Check sheet for the drawn part. Datum: minimum x, y, z corner. Units: mm. A direction names the side the tool comes from. Give positions to 0.01 mm unless a question says otherwise; leave off trailing zeros. Loops run counter-clockwise (first coordinate to the right, second up) from the corner with the lowest first, then second, coordinate; pieces in that order, holes last. Notation, with made-up numbers: (41, -15.5) - (54, -15.5) arc R19 cw to (54, 11.5) - close; hole circle Ø10 at (63, 46). An arc over 180 degrees is marked (long way). One line per item, written item: value. Start each with the question number.
1. Gauge pin test, flat ends, axial feed: pin 1 (5.5 mm diameter, centred on x = 6, z = 3.5, fed in from +Y); pin 2 (4 mm diameter, centred on x = 2.5, z = 47.5, fed in from +Y); pin 3 (5 mm diameter, centred on x = 6.5, y = 22.5, fed in from -Z); pin 4 (3 mm diameter, centred on y = 18, z = 25, fed in from +X). Record the tip position at first contact, or that the pin passes through.
2. Sectioned sample at A-A (z = 25). Record the cut outline in (x, y), plus the area to 3 significant figures.
3. Scan lines: L1, parallel to Y at x = 5, z = 25; L2, parallel to Y at x = 2, z = 39; L3, parallel to Y at x = 7, z = 2. Record each from-to range of solid material in increasing order. Write a range as [from, to].
4. Sectioned sample at C-C (y = 19.75). Record the cut outline in (x, z), plus the area to 3 significant figures.
5. Access from +Z, -Z, +X, -X, +Y, -Y to the whole of each face (thin tool, end or side, straight path). Record for the marked faces 1, 2 and 3.
6. Sectioned sample at D-D (z = 4.5). Record the cut outline in (x, y).
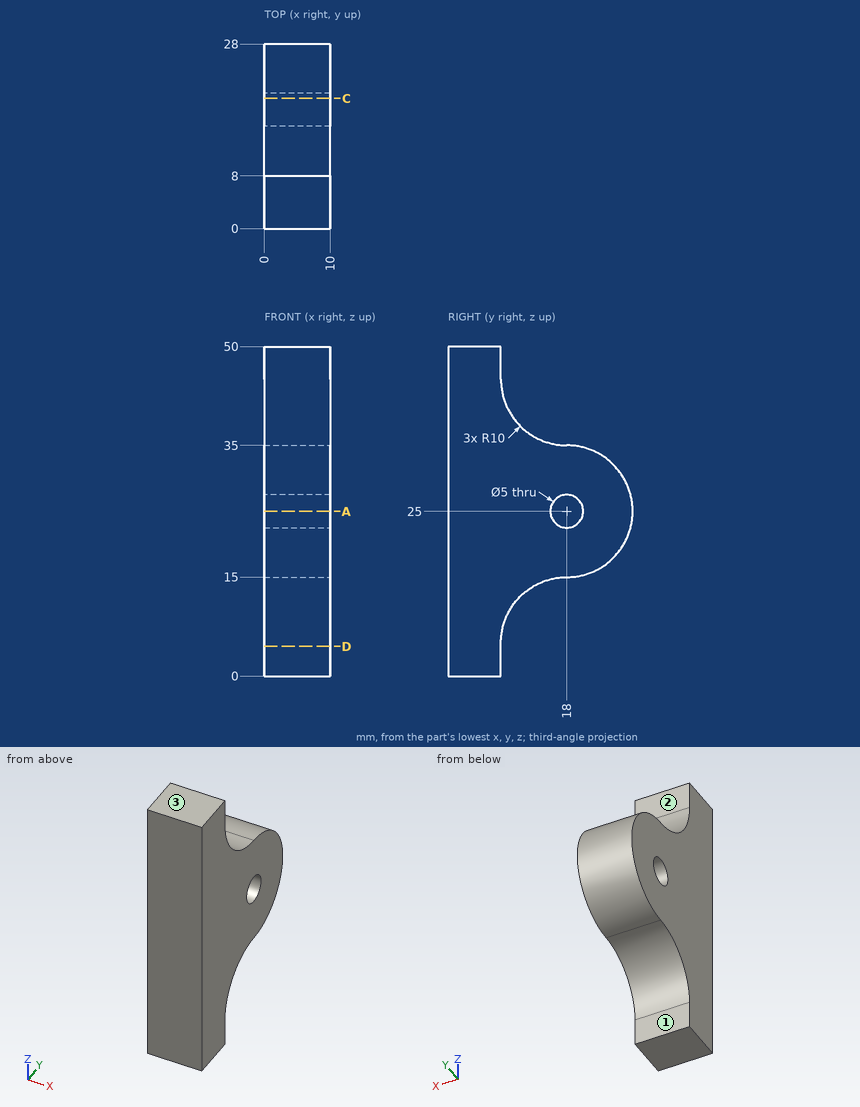
Results are:
1. pin 1: stops at y = 8.08
1. pin 2: stops at y = 8
1. pin 3: stops at z = 15.2
1. pin 4: passes through
2. outline: (0, 0) - (10, 0) - (10, 15.5) - (0, 15.5) - close; (0, 20.5) - (10, 20.5) - (10, 28) - (0, 28) - close
2. area: 230 mm^2
3. L1: y = [0, 15.5], [20.5, 28]
3. L2: y = [0, 10]
3. L3: y = [0, 8]
4. outline: (0, 15.15) - (10, 15.15) - (10, 23.21) - (0, 23.21) - close; (0, 26.79) - (10, 26.79) - (10, 34.85) - (0, 34.85) - close
4. area: 161 mm^2
5. face 1: -Z, +X, -X, +Y
5. face 2: +Z, +X, -X, +Y
5. face 3: +Z, +X, -X, +Y, -Y
6. outline: (0, 0) - (10, 0) - (10, 8) - (0, 8) - close
